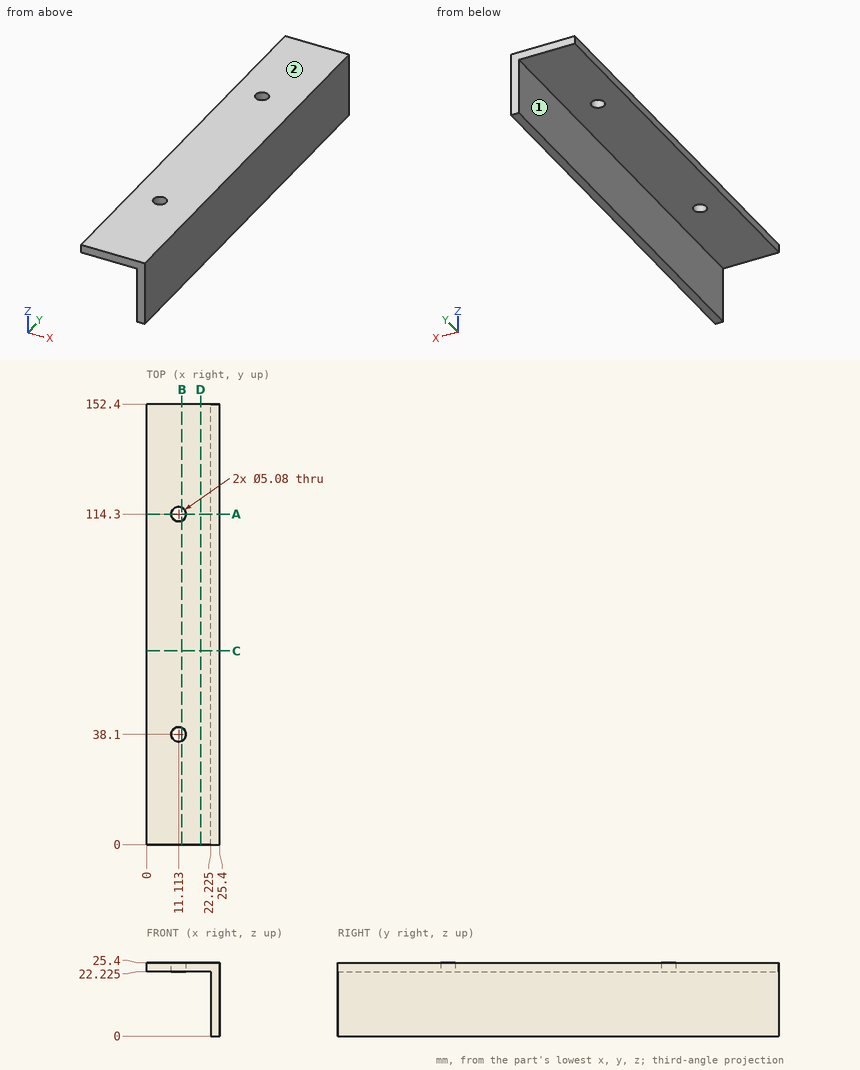
Design review of the part shown in the three views and the two pictorial views. Dimensions are in mm from the part's minimum x, y and z. A direction names the side the tool comes from. Round coordinates to 2 decimals unless told otherwise and drop trailing zeros. Loops run counter-clockwise (first coordinate to the right, second up) from the corner with the lowest first, then second, coordinate; pieces in that order, holes last.
(1) Wall thickness on line 1 along X through (y, z) = (114.3, 23.75); line 2 along Z through (x, y) = (10.75, 45) (1 decimal): over which ranges is each line inside the solid? List them lowest first.
Returned:
line 1: x = 0 to 8.57, 13.65 to 25.4
line 2: z = 22.2 to 25.4
(2) Clearance check with flat-ended pins moving along their axes: P1, Ø6, axis at x = 15.5, y = 35.5, coming from the -Z side (1 decimal); P2, Ø6.5, axis at y = 100.5, z = 10, coming from the -X side (1 decimal). State where each tip first meets the part, or that it passes through.
Returned:
P1: stops at z = 22.2
P2: stops at x = 22.2
(3) We need section B-B (x = 12.25). Give the boundary of the cut face in (y, z) (1 decimal), plus the area to 3 significant figures.
Returned:
outline: (0, 22.2) - (35.8, 22.2) - (35.8, 25.4) - (0, 25.4) - close; (40.4, 22.2) - (112, 22.2) - (112, 25.4) - (40.4, 25.4) - close; (116.6, 22.2) - (152.4, 22.2) - (152.4, 25.4) - (116.6, 25.4) - close
area: 455 mm2
(4) We need section D-D (x = 18.75). Give the boundary of the cut face in (y, z) (1 decimal).
Returned:
outline: (0, 22.2) - (152.4, 22.2) - (152.4, 25.4) - (0, 25.4) - close
(5) We need section A-A (y = 114.3). Give the boundary of the cut face in (x, z) (1 decimal), plus the area to 3 significant figures.
Returned:
outline: (0, 22.2) - (8.6, 22.2) - (8.6, 25.4) - (0, 25.4) - close; (13.7, 22.2) - (22.2, 22.2) - (22.2, 0) - (25.4, 0) - (25.4, 25.4) - (13.7, 25.4) - close
area: 135 mm2
(6) Tool access review of the marked faces 1 and 2: name each direction out of +Z, -Z, +X, -X, +Y, -Y from which nothing blocks a thin tool from reaching the whole face with its end or side.
Returned:
face 1: -Z, -X, +Y, -Y
face 2: +Z, +X, -X, +Y, -Y
(7) We need section C-C (y = 67). Give the boundary of the cut face in (x, z) (1 decimal).
Returned:
outline: (0, 22.2) - (22.2, 22.2) - (22.2, 0) - (25.4, 0) - (25.4, 25.4) - (0, 25.4) - close
